The listing builds one solid part. Answer for the finished solid, in the listing's coordinates (mm). Coordinates: 2 decimals unless noted, no trailing zeros. Order: outer loops, then holes, each group sorted by start corner. A loop starts at its lowest first (then second) coordinate and runs counter-clockwise, first axis right, second up. Notation, with made-up numbers: (-36.5, 7) -> (-25.5, 7) arc R11 cw to (-25.5, 16) -> close; hole circle Ø6 at (41, 89.5). An arc over 180 degrees is marked (long way). Write each question's results on one line, items separated by ' | '. Start each with the question number.
(1) Given pin 1 (3.5 mm diameter, centred on x = 4, y = 0, fed in from +Z); pin 2 (1.7 mm diameter, centred on x = 42, y = 0, fed in from +Z), each flat-ended and moving along its own axis, determine where each tip first touches the part or whether it passes through.
(2) The part is cut by section D-D, the plane y = 2.25. Give the vertices of the cut face in (x, z), then the cut area to 3 significant figures.
(3) The part is cut by section B-B, the plane z = -1.9. Give the vertices of the cut face in (x, y), then the cut area to 3 significant figures.
(4) The part is cut by section A-A, the plane y = 0. Count the separate pieces of the cut face and the enclosed holes in it, then the cut area to 3 significant figures.
(5) The part is cut by section C-C, the plane x = 38. Give the vertices of the cut face in (y, z).
(6) Straight lines are drawn through the part: L1, parallel to Y at x = 0, z = -1.95; L2, parallel to X at y = -2.75, z = -0.25; L3, parallel to X at y = 1, z = -1.2. For each, find the intervals that lie inside material, in ascending order.
(7) Determine the mould class of faces 1 (the face through (12, 0, 0)), 2 (the face through (-2.715, -3.699, -1.521)), 3 (the face through (39.45, 0.06, -1.52)) for opening direction X: +X half, -X half, draft (parallel to the pull), parting line (faces both ways), or undercut.
```python
from build123d import *

# Parameters (mm, degrees)
F0_W     = 6
F0_H     = 8
F0_W_2   = 36
F1_DEPTH = 3
F2_D     = 2.9
F4_D     = 2.3
F5_R     = 1


with BuildPart() as f1:
    # F0 (on Top) → F1 (new body)
    with BuildSketch(Plane.XY):
        Rectangle(F0_W, F0_H)
        with Locations((21, 0)):
            Rectangle(F0_W_2, F0_H)
        with Locations((42, 0)):
            Rectangle(F0_W, F0_H)
    extrude(amount=-F1_DEPTH)

    # F2 (through all)
    with Locations(Plane.XY):
        with Locations((0, 0), (4, 0), (38, 0), (42, 0)):
            Hole(F2_D / 2)

    # F4 (through all)
    with Locations(Plane.XZ.offset(4)):
        with Locations((9, 0), (15, 0), (21, 0), (27, 0), (33, 0)):
            Hole(F4_D / 2)

    # F5
    f5_edges = [f1.edges().sort_by_distance(p)[0] for p in [
        (-3, -4, -1.5),
        (45, -4, -1.5),
        (45, 4, -1.5),
        (-3, 4, -1.5),
    ]]
    fillet(f5_edges, radius=F5_R)


solid = f1.part
```
Established:
1) pin 1: stops at z = 0 | pin 2: passes through
2) outline: (-3, -3) -> (45, -3) -> (45, 0) -> (34.15, 0) arc R1.15 cw to (31.85, 0) -> (28.15, 0) arc R1.15 cw to (25.85, 0) -> (22.15, 0) arc R1.15 cw to (19.85, 0) -> (16.15, 0) arc R1.15 cw to (13.85, 0) -> (10.15, 0) arc R1.15 cw to (7.85, 0) -> (-3, 0) -> close | area: 134 mm^2
3) outline: (-3, -3) arc R1 ccw to (-2, -4) -> (44, -4) arc R1 ccw to (45, -3) -> (45, 3) arc R1 ccw to (44, 4) -> (-2, 4) arc R1 ccw to (-3, 3) -> close; hole circle Ø2.9 at (0, 0); hole circle Ø2.9 at (4, 0); hole circle Ø2.9 at (38, 0); hole circle Ø2.9 at (42, 0) | area: 357 mm^2
4) separate pieces: 5 | enclosed holes: 0 | area: 98.8 mm^2
5) outline: (-4, -3) -> (-1.45, -3) -> (-1.45, 0) -> (-4, 0) -> close; (1.45, -3) -> (4, -3) -> (4, 0) -> (1.45, 0) -> close
6) L1: y = -4 to -1.45, 1.45 to 4 | L2: x = -3 to 7.88, 10.12 to 13.88, 16.12 to 19.88, 22.12 to 25.88, 28.12 to 31.88, 34.12 to 45 | L3: x = -3 to -1.05, 1.05 to 2.95, 5.05 to 36.95, 39.05 to 40.95, 43.05 to 45
7) face 1: draft | face 2: -X half | face 3: undercut
